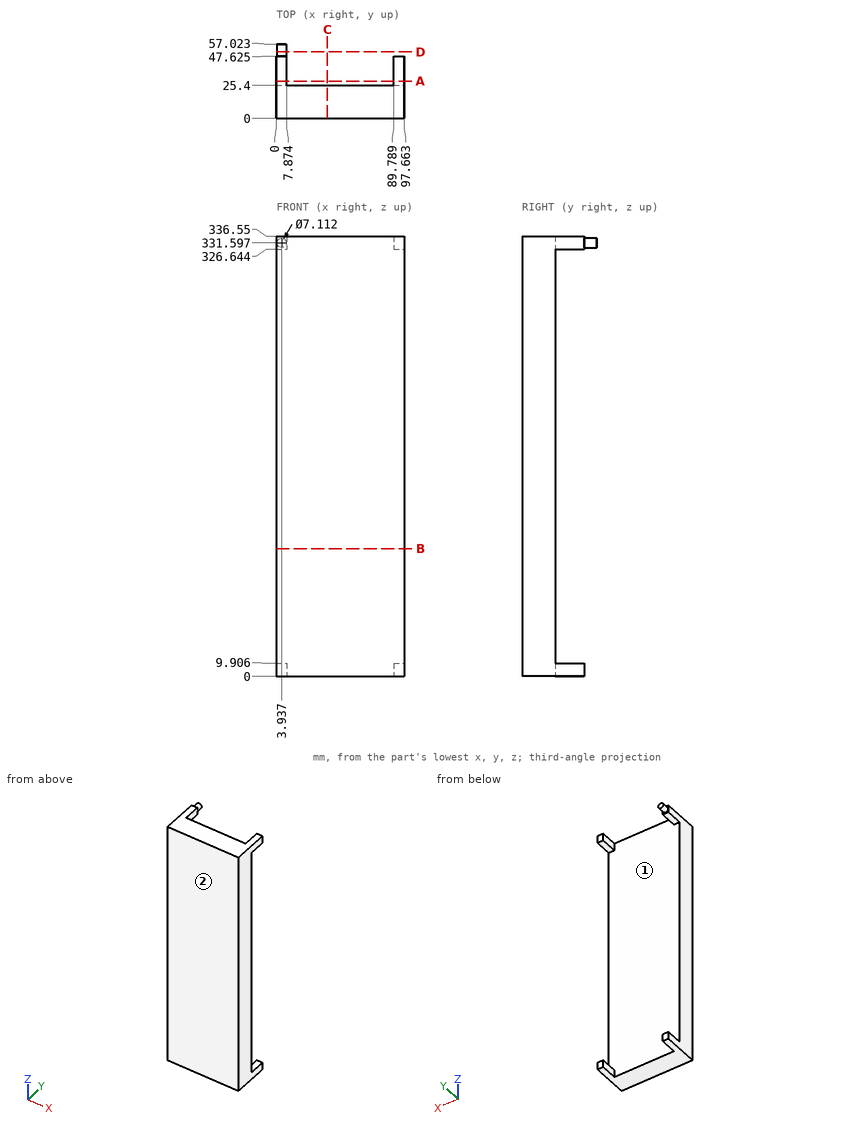
Answer from the drawing. Dimensions are ordinates in mm from the lowest x, y and z of the part. Coordinates: 2 decimals unless noted, no trailing zeros. Loops run counter-clockwise (first coordinate to the right, second up) from the corner with the lowest first, then second, coordinate; pieces in that order, holes last.
Q1. The part is cut by section C-C on x = 39. Write down the section's boundary in (y, z), and give its area (3 significant figures).
Q2. The mould has two halves that part along Z. Classify the marked faces 1 and 2: +Z half, -Z half, draft (parallel to the pull), parting line (faces both ways), or undercut.
Q3. Each of these flat-tipped pins is pushed along its axis until it touches: pin 1 Ø8.5 at (x, z) = (93, 334) entering from +Y (3 decimals); pin 2 Ø10 at (x, z) = (39, 237.5) entering from +Y. Where does it stop, or does it pass through?
Q4. Consider probe 1 along Y at (x, z) = (28, 40.5). Determine where the line is inside the solid, lowest interval first.
Q5. The part is cut by section A-A on y = 28.5. Write down the section's boundary in (x, z), and give its area (3 significant figures).
Q6. The part is cut by section B-B on z = 97.5. Write down the section's boundary in (x, y).
Q7. The part is cut by section D-D on y = 51. Write down the section's boundary in (x, z).
Results below:
1. outline: (0, 0) - (25.4, 0) - (25.4, 336.55) - (0, 336.55) - close
1. area: 8,550 mm2
2. face 1: undercut
2. face 2: draft
3. pin 1: stops at y = 47.625
3. pin 2: stops at y = 25.4
4. probe 1: y = 0 to 25.4
5. outline: (0, 0) - (7.87, 0) - (7.87, 9.91) - (0, 9.91) - close; (0, 326.64) - (7.87, 326.64) - (7.87, 336.55) - (0, 336.55) - close; (89.79, 0) - (97.66, 0) - (97.66, 9.91) - (89.79, 9.91) - close; (89.79, 326.64) - (97.66, 326.64) - (97.66, 336.55) - (89.79, 336.55) - close
5. area: 312 mm2
6. outline: (0, 0) - (97.66, 0) - (97.66, 25.4) - (0, 25.4) - close
7. outline: circle Ø7.11 at (3.94, 331.6)
